from build123d import *

# Parameters (mm, degrees)
SKETCH005_W       = 50
SKETCH005_H       = 40
PAD002_DEPTH      = 2
PAD003_DEPTH      = 50
SKETCH007_R       = 2.35
POCKET_DEPTH      = 15
POCKET_DEPTH_BACK = 100
SKETCH008_R       = 1.4
SKETCH008_R_2     = 1.75
POCKET001_DEPTH   = 5
FILLET004_R       = 2
FILLET005_R       = 2
FILLET006_R       = 2
FILLET007_R       = 2


with BuildPart() as part:
    # Sketch005 → Pad002 (new body)
    with BuildSketch(Plane.XZ):
        with Locations((74, -20)):
            Rectangle(SKETCH005_W, SKETCH005_H)
    extrude(amount=PAD002_DEPTH)

    # Sketch006 (on Face4 of Pad002) → Pad003 (join)
    with BuildSketch(Plane(origin=(99, 0, 0), x_dir=(0, 0, 1), z_dir=(1, 0, 0))):
        Polygon((-34.7, 0.798076), (-33.2, -1.8), (-26.8, -1.8), (-25.3, 0.798076), align=None)
        Polygon((-5.3, 0.798076), (-6.8, -1.8), (-13.2, -1.8), (-14.7, 0.798076), align=None)
    extrude(amount=-PAD003_DEPTH)

    # Sketch007 (on Face4 of Pad003) → Pocket (cut, two sides)
    with BuildSketch(Plane(origin=(0, 0, 0), x_dir=(1, 0, 0), z_dir=(0, 1, 0))) as pocket_sk:
        with Locations((85, 10)):
            Circle(SKETCH007_R)
    extrude(amount=-POCKET_DEPTH, mode=Mode.SUBTRACT)
    extrude(pocket_sk.sketch, amount=POCKET_DEPTH_BACK, mode=Mode.SUBTRACT)

    # Sketch008 (on Face5 of Pocket) → Pocket001 (cut)
    with BuildSketch(Plane.XZ.offset(2)):
        with Locations((58.268055, -30)):
            Circle(SKETCH008_R)
        with Locations((72, -30)):
            Circle(SKETCH008_R_2)
        with Locations((72, -10)):
            Circle(SKETCH008_R_2)
    extrude(amount=-POCKET001_DEPTH, mode=Mode.SUBTRACT)

    # Fillet004
    fillet004_edges = [part.edges().sort_by_distance(p)[0] for p in [
        (49, -1, -40),
    ]]
    fillet(fillet004_edges, radius=FILLET004_R)

    # Fillet005
    fillet005_edges = [part.edges().sort_by_distance(p)[0] for p in [
        (99, -1, -40),
    ]]
    fillet(fillet005_edges, radius=FILLET005_R)

    # Fillet006
    fillet006_edges = [part.edges().sort_by_distance(p)[0] for p in [
        (99, -1, 0),
    ]]
    fillet(fillet006_edges, radius=FILLET006_R)

    # Fillet007
    fillet007_edges = [part.edges().sort_by_distance(p)[0] for p in [
        (49, -1, 0),
    ]]
    fillet(fillet007_edges, radius=FILLET007_R)


solid = part.part
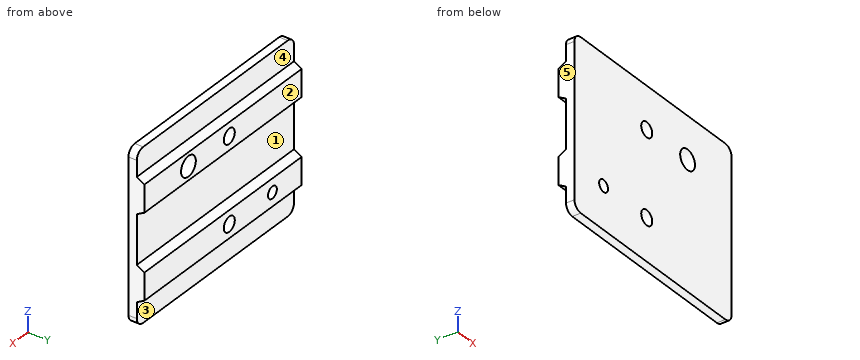
Part model, mm, in its own coordinate system. Face numbers are marked on the shaded views. A direction names the side the tool comes from. Round coordinates to 2 decimals unless told otherwise and drop trailing zeros. Write each loop counter-clockwise with the first axis right and the second up, starting at its lowest first coordinate (ties: lowest second). Pieces come first, ordered by that corner, then holes. Notation, with made-up numbers: M 13,62 L 37,62 A31 cw 37,97 Z; hole C -23,79.25 d5. An arc over 180 degrees is marked long. Return JSON: item names as keys, results as strings. Group by question number.
(1) Which spindle directions (+Z, -Z, +X, -X, +Y, -Y) get a long thin tool onto all of the face, cutting with end or side? Do the marked faces 3, 4 and 5. Say none if no direction does.
(2) Saw through at A-A on z = -30. Write the cut outline in (x, y), then the cut area to 3 significant figures.
(3) Saw through at B-B on x = 85. Write the cut outline in (y, z), then the cut area to 3 significant figures.
(4) Saw through at C-C on y = -1.4. Write the cut outline in (x, z).
(5) Two-plate mould, pull along Z, no slides. Class the marked faces 1 and 2: +Z half, -Z half, draft (parallel to the pull), parting line (faces both ways), or undercut.
(6) Pin check, flat tips, straight feed: pin 1 Ø1.5 at (x, y) = (68, 1.5) entering from +Z; pin 2 Ø9 at (x, z) = (81, -19.5) entering from +Y; pin 3 Ø4 at (x, z) = (85, -10) entering from -Y; pin 4 Ø10 at (x, z) = (59.5, -18.5) entering from +Y. Stop position of each tip, or through.
(7) Saw through at D-D on x = 72. Write the cut outline in (y, z).
(8) Drill centre lines: probe 1 along Z at (x, y) = (86, 1.15); probe 2 along Z at (x, y) = (72, 0.7); probe 3 along Y at (x, z) = (63, -34.5). Where is each one in solid material? Low to high.
Returned:
{
 "1": {"face 3": "-Z, +X, -X, +Y", "face 4": "+Z, +X, -X, +Y", "face 5": "+Z, -Z, -X, +Y, -Y"},
 "2": {"outline": "M 49,-2 L 56.87,-2 L 56.87,1.8 L 49,1.8 Z; M 59.67,-2 L 70.25,-2 L 70.25,1.8 L 59.67,1.8 Z; M 73.75,-2 L 99,-2 L 99,1.8 L 73.75,1.8 Z", "area": "166 mm²"},
 "3": {"outline": "M -2,-40 L 0,-40 L 0,-34.24 L 1.8,-33.2 L 1.8,-26.8 L 0,-25.76 L 0,-14.24 L 1.8,-13.2 L 1.8,-12.35 L -2,-12.35 Z; M -2,-7.65 L 1.8,-7.65 L 1.8,-6.8 L 0,-5.76 L 0,0 L -2,0 Z", "area": "88.9 mm²"},
 "4": {"outline": "M 49,-38 A2 ccw 51,-40 L 97,-40 A2 ccw 99,-38 L 99,-2 A2 ccw 97,0 L 51,0 A2 ccw 49,-2 Z; hole C 58.27,-30 d2.8; hole C 72,-30 d3.5; hole C 72,-10 d3.5; hole C 85,-10 d4.7"},
 "5": {"face 1": "undercut", "face 2": "draft"},
 "6": {"pin 1": "z = -6.19", "pin 2": "y = 0", "pin 3": "through", "pin 4": "y = 1.28"},
 "7": {"outline": "M -2,-40 L 0,-40 L 0,-34.24 L 1.8,-33.2 L 1.8,-31.75 L -2,-31.75 Z; M -2,-28.25 L 1.8,-28.25 L 1.8,-26.8 L 0,-25.76 L 0,-14.24 L 1.8,-13.2 L 1.8,-11.75 L -2,-11.75 Z; M -2,-8.25 L 1.8,-8.25 L 1.8,-6.8 L 0,-5.76 L 0,0 L -2,0 Z"},
 "8": {"probe 1": "-33.58 to -26.42, -13.58 to -12.13, -7.87 to -6.42", "probe 2": "-33.84 to -31.75, -28.25 to -26.16, -13.84 to -11.75, -8.25 to -6.16", "probe 3": "-2 to 0"}
}
